Work out the finished part from the listing and answer in its coordinate system (mm). Face numbers are marked on the shaded views. A direction names the side the tool comes from. Round coordinates to 2 decimals unless told otherwise and drop trailing zeros. Order: outer loops, then holes, each group sorted by start corner. A loop starts at its lowest first (then second) coordinate and runs counter-clockwise, first axis right, second up. Notation, with made-up numbers: M 86.5,25.5 L 138.5,25.5 A34 ccw 138.5,55.5 Z; hole C 37,35.25 d8. An arc over 180 degrees is marked long. Answer as a JSON object with one key per item and string values. Group by question number.
from build123d import *

# Parameters (mm, degrees)
CROQUIS1_W                       = 196
CROQUIS1_H                       = 190
SALIENTE_EXTRUIR1_DEPTH          = 3
CROQUIS3_R                       = 8
CORTAR_EXTRUIR1_DEPTH            = 50
REDONDEO1_R                      = 10
TALADRO_ROSCADO_M81_D            = 6.8
TALADRO_ROSCADO_M81_DEPTH        = 17
TALADRO_ROSCADO_M81_TIP          = 2.042926105
MATRIZL1_COUNT                   = 2
MATRIZL1_PITCH                   = 160
CROQUIS12_W                      = 150
CROQUIS12_H                      = 2
SALIENTE_EXTRUIR6_DEPTH          = 3
BRIDA_DE_ARISTA1_DEPTH           = 150
BRIDA_DE_ARISTA1_BEND_DEPTH      = 150
REDONDEO5_R                      = 8
TALADRO_DE_MARGEN_PARA_M51_D     = 5.5
TALADRO_DE_MARGEN_PARA_M51_DEPTH = 500
TALADRO_DE_MARGEN_PARA_M51_TIP   = 1.652366702
CORTAR_EXTRUIR2_DEPTH            = 230.834723225


# Sheet-metal steps are written as plain solids
with BuildPart() as part:
    # Croquis1 → Saliente-Extruir1 (new body)
    with BuildSketch(Plane.XY):
        Rectangle(CROQUIS1_W, CROQUIS1_H)
    extrude(amount=SALIENTE_EXTRUIR1_DEPTH)

    # Croquis3 → Cortar-Extruir1 (cut, symmetric)
    with BuildSketch(Plane.XY.offset(3)):
        with Locations((83, 0)):
            Circle(CROQUIS3_R)
        with Locations((-83, 0)):
            Circle(CROQUIS3_R)
    extrude(amount=CORTAR_EXTRUIR1_DEPTH, both=True, mode=Mode.SUBTRACT)

    # Redondeo1
    redondeo1_edges = [part.edges().sort_by_distance(p)[0] for p in [
        (-98, 95, 1.5),
        (98, 95, 1.5),
        (98, -95, 1.5),
        (-98, -95, 1.5),
    ]]
    fillet(redondeo1_edges, radius=REDONDEO1_R)

    # Taladro roscado M81
    with Locations(Plane(origin=(0, 0, 0), x_dir=(-1, 0, 0), z_dir=(0, 0, -1))):
        with Locations((-50, 20), (-50, -20), (50, 20), (50, -20)):
            Hole(TALADRO_ROSCADO_M81_D / 2, depth=TALADRO_ROSCADO_M81_DEPTH)
            with Locations((0, 0, -(TALADRO_ROSCADO_M81_DEPTH + TALADRO_ROSCADO_M81_TIP / 2))):  # 118° drill point
                Cone(0, TALADRO_ROSCADO_M81_D / 2, TALADRO_ROSCADO_M81_TIP, mode=Mode.SUBTRACT)

    # Croquis9 → Taladro de margen para M41 (revolve, cut)
    with BuildSketch(Plane(origin=(-83.5, -80, 0), x_dir=(0, 1, 0), z_dir=(1, 0, 0))):
        Polygon((0, 0), (0, 501.351936393), (2.25, 500), (2.25, 0), align=None)
    taladro_de_margen_para_m41 = revolve(axis=Axis((-83.5, -80, -6.35), (0, 0, 1)), mode=Mode.SUBTRACT)

    # MatrizL1: Taladro de margen para M41 ×2
    with Locations(*[(0, i * MATRIZL1_PITCH, 0) for i in range(1, MATRIZL1_COUNT)]):
        add(taladro_de_margen_para_m41, mode=Mode.SUBTRACT)

    # Simetría3: Taladro de margen para M41 across plane
    add(taladro_de_margen_para_m41.mirror(Plane(origin=(0, 0, 0), x_dir=(0, 0, 1), z_dir=(1, 0, 0))), mode=Mode.SUBTRACT)

    # Simetría3 copy 1 sketch → Simetría3 copy 1 (revolve, cut)
    with BuildSketch(Plane(origin=(83.5, 80, 0), x_dir=(0, 1, 0), z_dir=(-1, 0, 0))):
        Polygon((0, 0), (0, -501.351936393), (2.25, -500), (2.25, 0), align=None)
    revolve(axis=Axis((83.5, 80, -6.35), (0, 0, -1)), mode=Mode.SUBTRACT)

    # Croquis12 → Saliente-Extruir6 (add)
    with BuildSketch(Plane.XY.offset(3)):
        with Locations((0, 96)):
            Rectangle(CROQUIS12_W, CROQUIS12_H)
    saliente_extruir6 = extrude(amount=-SALIENTE_EXTRUIR6_DEPTH)

    # Simetría4: Saliente-Extruir6 across plane
    add(saliente_extruir6.mirror(Plane.ZX))

    # Brida de arista1 section (across the edge) → Brida de arista1 (add)
    with BuildSketch(Plane(origin=(-75, -100, 3), x_dir=(0, 1, 0), z_dir=(1, 0, 0))):
        with BuildLine():
            Line((-3, 3), (-3, 25))
            Line((-3, 25), (0, 25))
            Line((0, 25), (0, 3))
            ThreePointArc((0, 3), (0.878679656, 0.878679656), (3, 0))
            Line((3, 0), (3, -3))
            ThreePointArc((3, -3), (-1.242640687, -1.242640687), (-3, 3))
        make_face()
    extrude(amount=BRIDA_DE_ARISTA1_DEPTH)

    # Brida de arista1 section 2 (across the edge) → Brida de arista1 bend (add)
    with BuildSketch(Plane(origin=(75, 100, 3), x_dir=(0, -1, 0), z_dir=(-1, 0, 0))):
        with BuildLine():
            Line((-3, 3), (-3, 25))
            Line((-3, 25), (0, 25))
            Line((0, 25), (0, 3))
            ThreePointArc((0, 3), (0.878679656, 0.878679656), (3, 0))
            Line((3, 0), (3, -3))
            ThreePointArc((3, -3), (-1.242640687, -1.242640687), (-3, 3))
        make_face()
    extrude(amount=BRIDA_DE_ARISTA1_BEND_DEPTH)

    # Redondeo5
    redondeo5_edges = [part.edges().sort_by_distance(p)[0] for p in [
        (-75, -101.5, 28),
        (75, -101.5, 28),
        (75, 101.5, 28),
        (-75, 101.5, 28),
    ]]
    fillet(redondeo5_edges, radius=REDONDEO5_R)

    # Taladro de margen para M51
    with Locations(Plane(origin=(0, -103, 0), x_dir=(-1, 0, 0), z_dir=(0, -1, 0))):
        with Locations((67, -20), (-67, -20), (17, -20), (-17, -20)):
            Hole(TALADRO_DE_MARGEN_PARA_M51_D / 2, depth=TALADRO_DE_MARGEN_PARA_M51_DEPTH)
            with Locations((0, 0, -(TALADRO_DE_MARGEN_PARA_M51_DEPTH + TALADRO_DE_MARGEN_PARA_M51_TIP / 2))):  # 118° drill point
                Cone(0, TALADRO_DE_MARGEN_PARA_M51_D / 2, TALADRO_DE_MARGEN_PARA_M51_TIP, mode=Mode.SUBTRACT)

    # Croquis25 → Cortar-Extruir2 (cut, through all)
    with BuildSketch(Plane.XZ.offset(103)):
        with BuildLine():
            Line((67, 17), (17, 17))
            ThreePointArc((17, 17), (14, 20), (17, 23))
            Line((17, 23), (67, 23))
            ThreePointArc((67, 23), (70, 20), (67, 17))
        make_face()
        with BuildLine():
            Line((-17, 17), (-67, 17))
            ThreePointArc((-67, 17), (-70, 20), (-67, 23))
            Line((-67, 23), (-17, 23))
            ThreePointArc((-17, 23), (-14, 20), (-17, 17))
        make_face()
    extrude(amount=-CORTAR_EXTRUIR2_DEPTH, mode=Mode.SUBTRACT)


solid = part.part
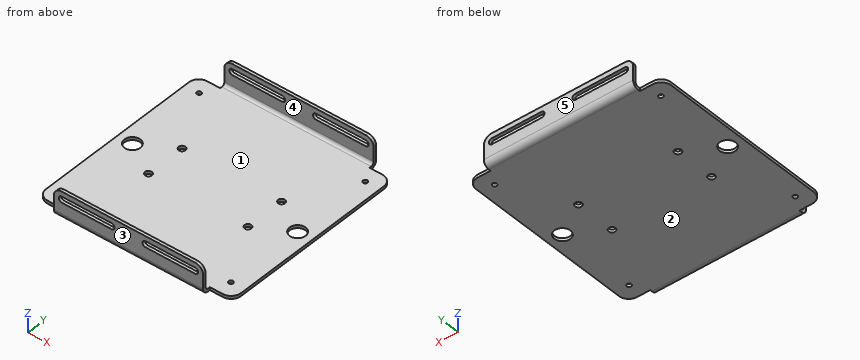
Item 1: Consider L1, parallel to X at y = 80, z = 1.55; L2, parallel to Y at x = -43.5, z = 25.5; L3, parallel to Y at x = -83, z = 0.9. Determine where each line is inside the solid, lowest interval first.
Item 2: Find section B-B (x = 26). Give the vertices of the cut face in (y, z).
Item 3: Find section C-C (x = 50). Give the vertices of the cut face in (y, z).
Item 4: Find section D-D (y = 71). Give the vertices of the cut face in (x, z), and give its area (3 significant figures).
Item 5: A tool of negligible diameter and unlimited length cuts with its end or side. For the marked faces 1 and 2, from which of +Z, -Z, +X, -X, +Y, -Y can it reach the whole face along a straight path? Write none if from no direction.
Item 6: Each of these flat-tipped pins is pushed along its axis until it touches: pin 1 (1.5 mm diameter, centred on x = -45.5, y = -101, fed in from -Z); pin 2 (5.5 mm diameter, centred on x = 50, y = -20, fed in from +Z); pin 3 (9 mm diameter, centred on y = -99, z = 8.5, fed in from -X); pin 4 (1 mm diameter, centred on x = -27, y = -71.5, fed in from -Z). Where does it stop, or does it pass through?
Item 7: The mould has two halves that part along Y. Classify the marked faces 3, 4 and 5: +Y half, -Y half, draft (parallel to the pull), parting line (faces both ways), or undercut.
Item 8: Find section A-A (y = 0). Give the vertices of the cut face in (x, z).
Responses:
{
 "1": {"L1": "x = -98 to -85.75, -81.25 to 81.25, 85.75 to 98", "L2": "y = -103 to -100, 100 to 103", "L3": "y = -95 to -82.19, -77.81 to -8, 8 to 77.81, 82.19 to 95"},
 "2": {"outline": "M -103,6 A6 ccw -97,0 L 97,0 A6 ccw 103,6 L 103,17 L 100,17 L 100,6 A3 cw 97,3 L -97,3 A3 cw -100,6 L -100,17 L -103,17 Z; M -103,23 L -100,23 L -100,28 L -103,28 Z; M 100,23 L 103,23 L 103,28 L 100,28 Z"},
 "3": {"outline": "M -103,6 A6 ccw -97,0 L -23.4,0 L -23.4,3 L -97,3 A3 cw -100,6 L -100,17 L -103,17 Z; M -103,23 L -100,23 L -100,28 L -103,28 Z; M -16.6,0 L 16.6,0 L 16.6,3 L -16.6,3 Z; M 23.4,0 L 97,0 A6 ccw 103,6 L 103,17 L 100,17 L 100,6 A3 cw 97,3 L 23.4,3 Z; M 100,23 L 103,23 L 103,28 L 100,28 Z"},
 "4": {"outline": "M -98,0 L 98,0 L 98,3 L -98,3 Z", "area": "588 mm^2"},
 "5": {"face 1": "+Z, +X, -X", "face 2": "-Z, +X, -X, +Y, -Y"},
 "6": {"pin 1": "stops at z = 0.96", "pin 2": "passes through", "pin 3": "stops at x = -75", "pin 4": "stops at z = 0"},
 "7": {"face 3": "-Y half", "face 4": "undercut", "face 5": "+Y half"},
 "8": {"outline": "M -98,0 L -91,0 L -91,3 L -98,3 Z; M -75,0 L 75,0 L 75,3 L -75,3 Z; M 91,0 L 98,0 L 98,3 L 91,3 Z"}
}
